```python
from build123d import *

# Parameters (mm, degrees)
SKETCH020_R             = 1.5
PAD013_DEPTH            = 15
PAD014_DEPTH            = 80
PAD015_DEPTH            = 80
SKETCH023_R             = 1.5
POCKET005_DEPTH         = 15
BODY003_PLACEMENT_ANGLE = 45


with BuildPart() as part:
    # Sketch020 → Pad013 (new body)
    with BuildSketch(Plane.XY):
        with BuildLine():
            ThreePointArc((59.887401, -16.046781), (62, 0), (59.887401, 16.046781))
            ThreePointArc((59.887401, 16.046781), (51.314187, 20.996528), (46.36444, 12.423314))
            ThreePointArc((43.66723, 6.1557), (46.103592, 8.821401), (46.36444, 12.423314))
            ThreePointArc((43.66723, 6.1557), (40, 0), (43.66723, -6.1557))
            ThreePointArc((46.36444, -12.423314), (46.103592, -8.821401), (43.66723, -6.1557))
            ThreePointArc((46.36444, -12.423314), (51.314187, -20.996528), (59.887401, -16.046781))
        make_face()
        with Locations((53.12592, 14.235047)):
            Circle(SKETCH020_R, mode=Mode.SUBTRACT)
        with Locations((53.12592, -14.235047)):
            Circle(SKETCH020_R, mode=Mode.SUBTRACT)
    extrude(amount=-PAD013_DEPTH)

    # Sketch021 → Pad014 (join)
    with BuildSketch(Plane.XY):
        with BuildLine():
            ThreePointArc((59.887401, -16.046781), (62, 0), (59.887401, 16.046781))
            ThreePointArc((59.887401, 16.046781), (51.314187, 20.996528), (46.36444, 12.423314))
            ThreePointArc((43.66723, 6.1557), (46.103592, 8.821401), (46.36444, 12.423314))
            ThreePointArc((43.66723, 6.1557), (40, 0), (43.66723, -6.1557))
            ThreePointArc((46.36444, -12.423314), (46.103592, -8.821401), (43.66723, -6.1557))
            ThreePointArc((46.36444, -12.423314), (51.314187, -20.996528), (59.887401, -16.046781))
        make_face()
        with BuildLine():
            ThreePointArc((57.95555, 15.529143), (51.831825, 19.064677), (48.296291, 12.940952))
            ThreePointArc((44.61945, 4.396929), (47.940703, 8.030817), (48.296291, 12.940952))
            ThreePointArc((44.61945, 4.396929), (42, 0), (44.61945, -4.396929))
            ThreePointArc((48.296291, -12.940952), (47.940703, -8.030817), (44.61945, -4.396929))
            ThreePointArc((48.296291, -12.940952), (51.831825, -19.064677), (57.95555, -15.529143))
            ThreePointArc((57.95555, -15.529143), (60, 0), (57.95555, 15.529143))
        make_face(mode=Mode.SUBTRACT)
    extrude(amount=-PAD014_DEPTH)

    # Sketch022 → Pad015 (join)
    with BuildSketch(Plane.XY):
        with BuildLine():
            ThreePointArc((55, -6), (61, 0), (55, 6))
            Line((55, 6), (47, 6))
            ThreePointArc((47, 6), (41, 0), (47, -6))
            Line((55, -6), (47, -6))
        make_face()
    extrude(amount=-PAD015_DEPTH)

    # Sketch023 → Pocket005 (cut)
    with BuildSketch(Plane.XY.offset(-80)):
        with Locations((47, 0)):
            Circle(SKETCH023_R)
        with Locations((55, 0)):
            Circle(SKETCH023_R)
    extrude(amount=POCKET005_DEPTH, mode=Mode.SUBTRACT)


with BuildPart() as part_1:
    # Body003 placement: moved
    add(part.part.moved(Location((0, 0, 25))).rotate(Axis((0, 0, 25), (0, 0, 1)), BODY003_PLACEMENT_ANGLE))


solid = part_1.part
```
Geometry check sheet. Reference: the model listing, model coordinates, mm. A direction names the side the tool comes from. Coordinates: 2 decimals unless noted, no trailing zeros. Answer as a JSON object with one key per item and string values.
1. Draft check along X on faces 1 (the cylindrical face through (38.567, 40.355, -47.605)), 2 (the cylindrical face through (26.39, 46.62, 17.6)), 3 (the cylindrical face through (21.516, 51.264, -14.44)), 4 (the cylindrical face through (44, 43.68, -14.44)). Enter one of: released by +X, released by -X, zero draft, split by the parting line, or undercut.
Answers below:
{"face 1": "undercut", "face 2": "undercut", "face 3": "split by the parting line", "face 4": "released by +X"}
2. Go/stop test with flat-tipped pins: pin 1 Ø10 at (y, z) = (31.5, -6) entering from -X; pin 2 Ø4 at (y, z) = (33, -9.5) entering from +X; pin 3 Ø0.9 at (x, y) = (39.5, 39.5) entering from -Z. Record where each tip stops, or that it passes through.
Answers below:
{"pin 1": "stops at x = 26.23", "pin 2": "stops at x = 53.69", "pin 3": "stops at z = -40"}
3. Scan lines: L1, parallel to Y at x = 38, z = -49; L2, parallel to Y at x = 34.5, z = -40.5; L3, parallel to X at y = 37, z = -26. Record each from-to range of solid material in increasing order.
Answers below:
{"L1": "y = 26.62 to 28.66, 29.51 to 37.68, 40.1 to 44.82, 46.43 to 48.99", "L2": "y = 26.35 to 32.43, 34.04 to 42.99, 49.09 to 51.51", "L3": "x = 26.75 to 44.59, 47.23 to 49.75"}
4. Tool access check on faces 5 (the cylindrical face through (50.04, 23.12, -22.04)), 6 (the cylindrical face through (48.324, 28.83, 17.605)). Record the directions out of +Z, -Z, +X, -X, +Y, -Y that give a thin tool (end or side, any length) a straight path to the whole face; none if there is none.
Answers below:
{"face 5": "-Z", "face 6": "+Z, -Z"}
